Check sheet for the modelled part. Datum: model origin and axes. Units: mm. A direction names the side the tool comes from. Round coordinates to 2 decimals unless told otherwise and drop trailing zeros. Write each loop counter-clockwise with the first axis right and the second up, starting at its lowest first coordinate (ties: lowest second). Pieces come first, ordered by that corner, then holes.
Item 1: Go/stop test with flat-tipped pins: pin 1 Ø4 at (x, y) = (29, 16) entering from -Z; pin 2 Ø4 at (x, y) = (33.94, 9.06) entering from +Z. Record where each tip stops, or that it passes through.
Item 2: Cross-section at B-B on y = 22.5. Enter the section's corners in (x, z).
Item 3: Release check for a two-part mould opening along Y. For faces 4 (the conical face through (33.88, 36.37, 15.76)), 5 (the flat face through (21, 45, 17)), 6 (the flat face through (21, 0, 17)), 7 (the flat face through (0, 22, 17)) record: +Y half, -Y half, draft (parallel to the pull), parting line (faces both ways), or undercut.
Item 4: Material ranges on line 1 (Y direction, x = 35, z = 4); line 2 (Y direction, x = 20, z = 15); line 3 (Z direction, x = 21.5, y = 42.5), recorded low to high.
Item 5: Cross-section at A-A on x = 20.5. Enter the section's corners in (y, z), plus the area to 3 significant figures.
Item 6: Tool access check on faces 1 (the cylindrical face through (29.325, 39.137, 21.969)), 2 (the cylindrical face through (4.68, 9.82, 25.38)), 3 (the flat face through (35, 28, 34)). Record the directions out of +Z, -Z, +X, -X, +Y, -Y that give a thin tool (end or side, any length) a straight path to the whole face; none if there is none.
Item 7: Cross-section at D-D on z = 26.5. Enter the section's corners in (x, y), plus the area to 3 significant figures.
Item 8: Cross-section at C-C on z = 11. Enter the section's corners in (x, y).
from build123d import *

# Parameters (mm, degrees)
SZKIC1_W                       = 42
SZKIC1_H                       = 45
SZKIC1_R                       = 14
DODANIE_WYCI_GNI_CIE1_DEPTH    = 34
SFAZOWANIE1_SIZE               = 1
OTW_R_GWINTOWANY_M6X1_01_D     = 5
OTW_R_GWINTOWANY_M6X1_01_DEPTH = 17
OTW_R_GWINTOWANY_M6X1_01_TIP   = 1.502151548
OTW_R_GWINTOWANY_M5X0_82_D     = 4.2
OTW_R_GWINTOWANY_M5X0_82_DEPTH = 25
OTW_R_GWINTOWANY_M5X0_82_TIP   = 1.2618073


with BuildPart() as part:
    # Szkic1 → Dodanie-wyciągnięcie1 (new body)
    with BuildSketch(Plane.XY):
        with Locations((21, 22.5)):
            Rectangle(SZKIC1_W, SZKIC1_H)
        with Locations((20.5, 22.5)):
            Circle(SZKIC1_R, mode=Mode.SUBTRACT)
    extrude(amount=DODANIE_WYCI_GNI_CIE1_DEPTH)

    # Sfazowanie1
    sfazowanie1_edges = [part.edges().sort_by_distance(p)[0] for p in [
        (6.5, 22.5, 0),
        (6.5, 22.5, 34),
    ]]
    chamfer(sfazowanie1_edges, length=SFAZOWANIE1_SIZE)

    # Otwór gwintowany M6x1.01
    with Locations(Plane.XY.offset(34)):
        with Locations((33.935028843, 35.935028843), (7.064971157, 35.935028843), (7.064971157, 9.064971157), (33.935028843, 9.064971157)):
            Hole(OTW_R_GWINTOWANY_M6X1_01_D / 2, depth=OTW_R_GWINTOWANY_M6X1_01_DEPTH)
            with Locations((0, 0, -(OTW_R_GWINTOWANY_M6X1_01_DEPTH + OTW_R_GWINTOWANY_M6X1_01_TIP / 2))):  # 118° drill point
                Cone(0, OTW_R_GWINTOWANY_M6X1_01_D / 2, OTW_R_GWINTOWANY_M6X1_01_TIP, mode=Mode.SUBTRACT)

    # Otwór gwintowany M5x0.82
    with Locations(Plane(origin=(42, 0, 0), x_dir=(0, 0, -1), z_dir=(1, 0, 0))):
        with Locations((-21, 41), (-4, 41), (-4, 4), (-21, 4)):
            Hole(OTW_R_GWINTOWANY_M5X0_82_D / 2, depth=OTW_R_GWINTOWANY_M5X0_82_DEPTH)
            with Locations((0, 0, -(OTW_R_GWINTOWANY_M5X0_82_DEPTH + OTW_R_GWINTOWANY_M5X0_82_TIP / 2))):  # 118° drill point
                Cone(0, OTW_R_GWINTOWANY_M5X0_82_D / 2, OTW_R_GWINTOWANY_M5X0_82_TIP, mode=Mode.SUBTRACT)


solid = part.part
Response values:
1. pin 1: passes through
1. pin 2: stops at z = 16.7
2. outline: (0, 0) - (5.5, 0) - (6.5, 1) - (6.5, 33) - (5.5, 34) - (0, 34) - close; (34.5, 1) - (35.5, 0) - (42, 0) - (42, 34) - (35.5, 34) - (34.5, 33) - close
3. face 4: undercut
3. face 5: +Y half
3. face 6: -Y half
3. face 7: draft
4. line 1: y = 0 to 1.9, 6.1 to 38.9, 43.1 to 45
4. line 2: y = 0 to 8.51, 36.49 to 45
4. line 3: z = 0 to 2.53, 5.47 to 19.53, 22.47 to 34
5. outline: (0, 0) - (7.5, 0) - (8.5, 1) - (8.5, 33) - (7.5, 34) - (0, 34) - close; (36.5, 1) - (37.5, 0) - (45, 0) - (45, 34) - (37.5, 34) - (36.5, 33) - close; hole circle Ø4.2 at (4, 4); hole circle Ø4.2 at (4, 21); hole circle Ø4.2 at (41, 4); hole circle Ø4.2 at (41, 21)
5. area: 521 mm2
6. face 1: +X
6. face 2: +Z
6. face 3: +Z, +X, -X, +Y, -Y
7. outline: (0, 0) - (42, 0) - (42, 45) - (0, 45) - close; hole circle Ø5 at (7.06, 9.06); hole circle Ø5 at (7.06, 35.94); hole circle Ø28 at (20.5, 22.5); hole circle Ø5 at (33.94, 9.06); hole circle Ø5 at (33.94, 35.94)
7. area: 1,200 mm2
8. outline: (0, 0) - (42, 0) - (42, 45) - (0, 45) - close; hole circle Ø28 at (20.5, 22.5)
